Part model, mm, in its own coordinate system. Give positions to 0.01 mm unless a question says otherwise; leave off trailing zeros. Write each loop counter-clockwise with the first axis right and the second up, starting at its lowest first coordinate (ties: lowest second). Pieces come first, ordered by that corner, then holes. Notation, with made-up numbers: (-33, 38) - (-18, 38) arc R12 ccw to (-18, 49) - close; hole circle Ø8 at (-28, 12). An arc over 180 degrees is marked (long way). Answer in a Markdown table with one row per item. Add a question column.
1. Pull direction Y, two halves, no side cores. Call faces 1 (the flat face through (-5, 3, 0)), 2 (the flat face through (-5, 6.35, -22)), 3 (the flat face through (-5, 0, -22)): released by +Y, released by -Y, zero draft, split by the parting line, or undercut.
2. Probe line 1 along Z through (x, y) = (-5.5, 3.5); line 2 along Z through (x, y) = (-6.75, 2); line 3 along X through (y, z) = (1, -3.5). List the from-to ranges inside material, lowest first.
3. Drop a flat-ended pin along its axis: pin 1 Ø2 at (x, z) = (-5.52, -40.16) entering from -Y. Give the stop position or say it passes through.
4. Band-saw the part on B-B on y = 4.25. Write the cut outline in (x, z), plus the area to 3 significant figures.
5. Band-saw the part on A-A on x = -6. Write the cut outline in (y, z).
Autodesk Inventor part; units mm, degrees
ref_plane "YZ Plane" through (0, 0, 0) normal (1, 0, 0) x (0, 1, 0)
ref_plane "XZ Plane" through (0, 0, 0) normal (0, 1, 0) x (-1, 0, 0)
ref_plane "XY Plane" through (0, 0, 0) normal (0, 0, 1) x (1, 0, 0)
sketch "Sketch1" plane through (0, 0, 0) normal (0, 1, 0) x (-1, 0, 0)
  line L0 (-0.8262, 0) -> (11.8738, 0)
  line L1 (11.8738, 0) -> (11.8738, -44.45)
  line L2 (11.8738, -44.45) -> (-0.8262, -44.45)
  line L3 (-0.8262, -44.45) -> (-0.8262, 0)
  point P0 (0, 0)
  dimension "d0" = 44.45
  dimension "d1" = 12.7
extrude "Plate1" add sketch "Sketch1" along normal blind 6.35
sketch "Sketch2" plane through (0, 6.35, 0) normal (0, 1, 0) x (1, 0, 0)
  line L0 (0.8262, 0) -> (-11.8738, 0)
  line L1 (0.8262, 44.45) -> (0.8262, 0)
  point P0 (0, 0)
  point P1 (-5.5238, 4.5974)
  point P2 (-5.5238, 40.1574)
  dimension "d4" = 35.56
  dimension "d5" = 4.5974
  dimension "d6" = 6.35
  dimension "d7" = 6.35
hole "Hole1" at (-5.5238, 6.35, -4.5974) at (-5.5238, 6.35, -40.1574) direction (0, -1, 0) diameter 3.2766 end through all
equation "\"d13\" = Thickness"
equation "\"d2\" = Thickness"
equation "\"BendRadius\" = Thickness"
equation "\"BendReliefWidth\" = Thickness"
equation "\"BendReliefDepth\" = 0.5 * Thickness"
equation "\"CornerReliefSize\" = 4 * Thickness"
equation "\"MinimumRemnant\" = 2 * Thickness"
equation "\"TransitionRadius\" = BendRadius"
equation "\"JacobiRadiusSize\" = BendRadius"
equation "\"GapSize\" = Thickness"
properties part number "servo hold down"
Values:
| question | item | result |
|---|---|---|
| 1 | face 1 | zero draft |
| 1 | face 2 | released by +Y |
| 1 | face 3 | released by -Y |
| 2 | line 1 | z = -44.45 to -41.8, -38.52 to -6.24, -2.96 to 0 |
| 2 | line 2 | z = -44.45 to -41.24, -39.07 to -5.68, -3.51 to 0 |
| 2 | line 3 | x = -11.87 to -6.74, -4.31 to 0.83 |
| 3 | pin 1 | passes through |
| 4 | outline | (-11.87, -44.45) - (0.83, -44.45) - (0.83, 0) - (-11.87, 0) - close; hole circle Ø3.28 at (-5.52, -40.16); hole circle Ø3.28 at (-5.52, -4.6) |
| 4 | area | 548 mm² |
| 5 | outline | (0, -44.45) - (6.35, -44.45) - (6.35, -41.72) - (0, -41.72) - close; (0, -38.59) - (6.35, -38.59) - (6.35, -6.16) - (0, -6.16) - close; (0, -3.03) - (6.35, -3.03) - (6.35, 0) - (0, 0) - close |
